Read the model definition and answer for the solid it produces. Units are mm, in the model's axes. Round coordinates to 2 decimals unless told otherwise and drop trailing zeros. Order: outer loops, then holes, each group sorted by start corner. A loop starts at its lowest first (then second) coordinate and runs counter-clockwise, first axis right, second up. Notation, with made-up numbers: (-25, 33) -> (17, 33) arc R26 ccw to (17, 71) -> close; hole circle Ø8 at (-15.5, 52.5). An arc over 180 degrees is marked (long way). One line per item, written item: value. Start each with the question number.
1. A flat-ended cylindrical pin translates along its axis: pin 1 Ø1 at (y, z) = (-57.5, 2) entering from -X. Find the tip coordinate at first contact, or state that the pin passes through.
2. Section A-A (x = 0) is taken. Give the vertices of the cut face in (y, z).
3. Consider line 1 (X direction, y = 0, z = 1.5); line 2 (Y direction, x = -1.25, z = 2.65); line 3 (Y direction, x = 1, z = 2.85). Determine where each line is inside the solid, lowest interval first.
4. Section D-D (y = -5) is taken. Give the vertices of the cut face in (x, z), then the cut area to 3 significant figures.
5. The mould has two halves that part along Y. Classify faces 1 (the face through (0, -35, 3)), 2 (the face through (-4.035, -34.417, 1.479)): released by +Y, released by -Y, zero draft, split by the parting line, or undercut.
6. Section B-B (z = 1.3) is taken. Give the vertices of the cut face in (x, y), then the cut area to 3 significant figures.
7. Section C-C (y = -29) is taken. Give the vertices of the cut face in (x, z), then the cut area to 3 significant figures.
Autodesk Inventor part; units mm, degrees
ref_plane "YZ Plane" through (0, 0, 0) normal (1, 0, 0) x (0, 1, 0)
ref_plane "XZ Plane" through (0, 0, 0) normal (0, 1, 0) x (-1, 0, 0)
ref_plane "XY Plane" through (0, 0, 0) normal (0, 0, 1) x (1, 0, 0)
sketch "スケッチ1" plane through (0, 0, 0) normal (0, 0, 1) x (1, 0, 0)
  line L0 (0, 0) -> (0, -70) construction
  arc A0 (0, -5) -> (4.9881, -0.3446) centre (0, 0) ccw construction
  arc A1 (0, -64) -> (-5.9715, -69.4162) centre (0, -70) ccw construction
  arc A2 (-5.9715, -69.4162) -> (-4.9881, -0.3446) centre (-419.5607, -28.9848) ccw
  arc A3 (4.9881, -0.3446) -> (5.9715, -69.4162) centre (419.5607, -28.9848) ccw
  arc A4 (-4.9881, -0.3446) -> (0, -5) centre (0, 0) ccw construction
  arc A5 (4.9881, -0.3446) -> (-4.9881, -0.3446) centre (0, 0) ccw
  arc A6 (5.9715, -69.4162) -> (0, -64) centre (0, -70) ccw construction
  arc A7 (-5.9715, -69.4162) -> (5.9715, -69.4162) centre (0, -70) ccw
  line L1 (4, 0) -> (4, -70) construction
  dimension "d0" = 70
  dimension "d1" = 5
  dimension "d2" = 6
  dimension "d4" = 4
extrude "押し出し1" add sketch "スケッチ1" along normal blind 3
hole "穴1" at (0, 0, 0) at (0, -70, 0) direction (0, 0, 1) diameter 4 end through all
properties part number "COXA_ROLL_LONG-LINK"
Answer:
1. pin 1: x = -5.01
2. outline: (-76, 0) -> (-72, 0) -> (-72, 3) -> (-76, 3) -> close; (-68, 0) -> (-2, 0) -> (-2, 3) -> (-68, 3) -> close; (2, 0) -> (5, 0) -> (5, 3) -> (2, 3) -> close
3. line 1: -5 to -2, 2 to 5
3. line 2: -75.87 to -71.56, -68.44 to -1.56, 1.56 to 4.84
3. line 3: -75.92 to -71.73, -68.27 to -1.73, 1.73 to 4.9
4. outline: (-4.69, 0) -> (4.69, 0) -> (4.69, 3) -> (-4.69, 3) -> close
4. area: 28.2 mm^2
5. face 1: zero draft
5. face 2: undercut
6. outline: (-5.97, -69.42) arc R6 ccw (long way) to (5.97, -69.42) arc R415.56 cw to (4.99, -0.34) arc R5 ccw (long way) to (-4.99, -0.34) arc R415.56 cw to start; hole circle Ø4 at (0, -70); hole circle Ø4 at (0, 0)
6. area: 706 mm^2
7. outline: (-4, 0) -> (4, 0) -> (4, 3) -> (-4, 3) -> close
7. area: 24.0 mm^2
